Work out the finished part from the listing and answer in its coordinate system (mm). Face numbers are marked on the shaded views. A direction names the side the tool comes from. Round coordinates to 2 decimals unless told otherwise and drop trailing zeros. Write each loop counter-clockwise with the first axis right and the second up, starting at its lowest first coordinate (ties: lowest second). Pieces come first, ordered by that corner, then holes.
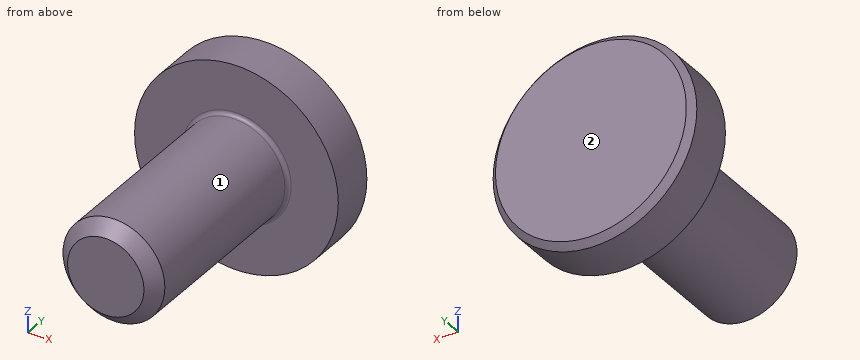
from build123d import *

# Parameters (mm, degrees)
SKETCH1_R           = 4
BOSS_EXTRUDE1_DEPTH = 16
SKETCH2_R           = 8
BOSS_EXTRUDE2_DEPTH = 4
CHAMFER1_SIZE       = 1
CHAMFER2_SIZE       = 0.5
FILLET1_R           = 0.3


with BuildPart() as part:
    # Sketch1 → Boss-Extrude1 (new body)
    with BuildSketch(Plane(origin=(0, 0, 0), x_dir=(1, 0, 0), z_dir=(0, 1, 0))):
        Circle(SKETCH1_R)
    extrude(amount=-BOSS_EXTRUDE1_DEPTH)

    # Sketch2 → Boss-Extrude2 (add)
    with BuildSketch(Plane(origin=(0, 0, 0), x_dir=(1, 0, 0), z_dir=(0, 1, 0))):
        Circle(SKETCH2_R)
    extrude(amount=BOSS_EXTRUDE2_DEPTH)

    # Chamfer1
    chamfer1_edges = [part.edges().sort_by_distance(p)[0] for p in [
        (-4, -16, 0),
    ]]
    chamfer(chamfer1_edges, length=CHAMFER1_SIZE)

    # Chamfer2
    chamfer2_edges = [part.edges().sort_by_distance(p)[0] for p in [
        (-8, 4, 0),
    ]]
    chamfer(chamfer2_edges, length=CHAMFER2_SIZE)

    # Fillet1
    fillet1_edges = [part.edges().sort_by_distance(p)[0] for p in [
        (-4, 0, 0),
    ]]
    fillet(fillet1_edges, radius=FILLET1_R)


solid = part.part
Q1. Find section B-B (z = 0). Determine the outline of the cut face in (x, y).
Q2. Find the intervals of material crossed by L1, parallel to Y at x = 4.5, z = -4.25; L2, parallel to X at y = -4.25, z = -2.5; L3, parallel to Y at x = -3.25, z = 1.5, in increasing order.
Q3. Find section C-C (y = -1.5). Determine the outline of the cut face in (x, z), plus the area to 3 significant figures.
Q4. Find section A-A (x = 0). Determine the outline of the cut face in (y, z).
Q5. Given pin 1 (4 mm diameter, centred on y = -4, z = -1, fed in from +X); pin 2 (5 mm diameter, centred on y = 1, z = -3.5, fed in from +X); pin 3 (2 mm diameter, centred on x = 4.5, z = -2.5, fed in from -Y), each flat-ended and moving along its own axis, determine where each tip first touches the part or whether it passes through.
Q6. Find section D-D (y = 1.75). Determine the outline of the cut face in (x, z), plus the area to 3 significant figures.
Q7. A tool of negligible diameter and unlimited length cuts with its end or side. For the marked faces 1 and 2, from which of +Z, -Z, +X, -X, +Y, -Y can it reach the whole face along a straight path? Write none if from no direction.
Report:
1. outline: (-8, 0) - (-4.3, 0) arc R0.3 cw to (-4, -0.3) - (-4, -15) - (-3, -16) - (3, -16) - (4, -15) - (4, -0.3) arc R0.3 cw to (4.3, 0) - (8, 0) - (8, 3.5) - (7.5, 4) - (-7.5, 4) - (-8, 3.5) - close
2. L1: y = 0 to 4
2. L2: x = -3.12 to 3.12
2. L3: y = -15.42 to 4
3. outline: circle Ø8 at (0, 0)
3. area: 50.3 mm2
4. outline: (-16, -3) - (-15, -4) - (-0.3, -4) arc R0.3 cw to (0, -4.3) - (0, -8) - (3.5, -8) - (4, -7.5) - (4, 7.5) - (3.5, 8) - (0, 8) - (0, 4.3) arc R0.3 cw to (-0.3, 4) - (-15, 4) - (-16, 3) - close
5. pin 1: stops at x = 4
5. pin 2: stops at x = 7.94
5. pin 3: stops at y = -0.04
6. outline: circle Ø16 at (0, 0)
6. area: 201 mm2
7. face 1: -Y
7. face 2: +Z, -Z, +X, -X, +Y
